from build123d import *

# Parameters (mm, degrees)
F1_DEPTH = 558.8


with BuildPart() as f1:
    # F0 (on Right) → F1 (new body)
    with BuildSketch(Plane.YZ):
        with BuildLine():
            Line((-203.2, 0), (0, 0))
            Line((0, 0), (24.326557, 0))
            Line((24.326557, 0), (143.169588, 266.830928))
            Line((143.169588, 266.830928), (-50.079897, 441.292268))
            Line((-50.079897, 441.292268), (-339.430412, 120.780928))
            Line((-339.430412, 120.780928), (-207.455155, 1.636598))
            ThreePointArc((-207.455155, 1.636598), (-205.479517, 0.423255), (-203.2, 0))
        make_face()
    extrude(amount=F1_DEPTH)


solid = f1.part
Geometry: final body of the model. Coordinates: model frame, mm. Round coordinates to 2 decimals unless told otherwise and drop trailing zeros. Loops run counter-clockwise (first coordinate to the right, second up) from the corner with the lowest first, then second, coordinate; pieces in that order, holes last. Notation, with made-up numbers: (79.25, -10) - (88.25, -10) arc R26 ccw to (88.25, 5) - close; hole circle Ø9 at (89.25, 53.5). An arc over 180 degrees is marked (long way). Write each question's results on one line, items separated by ' | '. Start each with the question number.
1) First-contact query: P1, Ø5, axis at x = 347, z = 293, coming from the +Y side; P2, Ø3, axis at x = 229.5, y = -161, coming from the +Z side; P3, Ø3, axis at x = 363, y = -98, coming from the +Z side. Flat tips, straight axial feed; report the tip coordinate or a pass-through.
2) Cut plane B-B on y = -173. Return loops of the section in (x, z).
3) Cut plane C-C on y = -266. Return loops of the section in (x, z), then the cut area to 3 significant figures.
4) Line query: probe 1 along Y at (x, z) = (261.5, 53); probe 2 along Y at (x, z) = (214, 144); probe 3 along Z at (x, y) = (105.5, 87). Output: solid intervals per line, ascending. Write a range as [from, to].
5) Cut plane A-A on x = 377.5. Return loops of the section in (y, z).
Verdict:
1) P1: stops at y = 116.95 | P2: stops at z = 320.09 | P3: stops at z = 389.87
2) outline: (0, 0) - (558.8, 0) - (558.8, 305.13) - (0, 305.13) - close
3) outline: (0, 54.49) - (558.8, 54.49) - (558.8, 202.12) - (0, 202.12) - close | area: 82,500 mm2
4) probe 1: y = [-264.35, 47.93] | probe 2: y = [-318.47, 88.46] | probe 3: z = [140.72, 317.54]
5) outline: (-339.43, 120.78) - (-207.46, 1.64) arc R6.35 ccw to (-203.2, 0) - (24.33, 0) - (143.17, 266.83) - (-50.08, 441.29) - close
